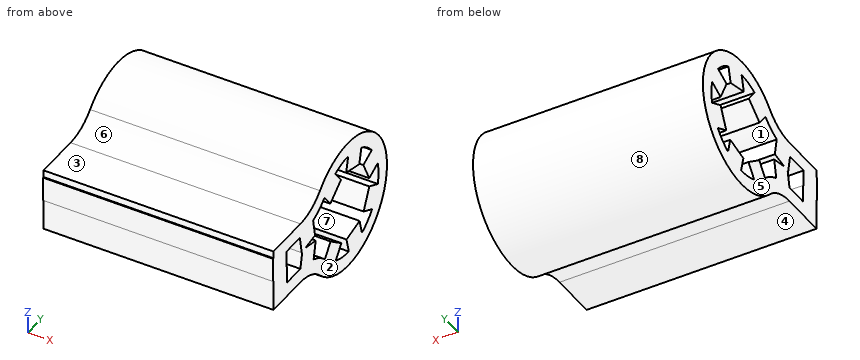
```python
from build123d import *

# Parameters (mm, degrees)
BOSS_EXTRUDE1_DEPTH = 5
BOSS_EXTRUDE2_DEPTH = 10
CRVPATTERN1_START   = -5
CRVPATTERN1_DEPTH   = 10


# Read off the part's stored shape, not the designer's step: CrvPattern1
with BuildPart() as part:
    # Sketch1 → Boss-Extrude1 (new, symmetric)
    with BuildSketch(Plane(origin=(0, 0, 0), x_dir=(0, 0, -1), z_dir=(1, 0, 0))):
        with BuildLine():
            Line((-0.74, -4.899518381), (-0.74, -3.529518381))
            ThreePointArc((-0.74, -3.529518381), (-0.951991552, -2.495045015), (-1.553790984, -1.627339417))
            ThreePointArc((-1.553790984, -1.627339417), (0, 2.25), (1.553790984, -1.627339417))
            ThreePointArc((1.553790984, -1.627339417), (0.951991552, -2.495045015), (0.74, -3.529518381))
            Line((0.74, -3.529518381), (0.74, -4.899518381))
            Line((0.74, -4.899518381), (0.74, -5.529518381))
            Line((0.74, -5.529518381), (1.37, -5.529518381))
            Line((1.37, -5.529518381), (1.37, -3.529518381))
            ThreePointArc((1.37, -3.529518381), (1.531210305, -2.74284662), (1.988852459, -2.082994454))
            ThreePointArc((1.988852459, -2.082994454), (0, 2.88), (-1.988852459, -2.082994454))
            ThreePointArc((-1.988852459, -2.082994454), (-1.531210305, -2.74284662), (-1.37, -3.529518381))
            Line((-1.37, -3.529518381), (-1.37, -5.529518381))
            Line((-1.37, -5.529518381), (-0.74, -5.529518381))
            Line((-0.74, -5.529518381), (-0.74, -4.899518381))
        make_face()
    extrude(amount=BOSS_EXTRUDE1_DEPTH, both=True)

    # Sketch2 → Boss-Extrude2 (add)
    with BuildSketch(Plane(origin=(5, 0, 0), x_dir=(0, 0, -1), z_dir=(1, 0, 0))):
        Polygon((0.74, -5.529518381), (-0.01, -5.529518381), (-0.01, -4.529518381), (1.055, -4.529518381), (1.055, -5.529518381), align=None)
    extrude(amount=-BOSS_EXTRUDE2_DEPTH)

    # CrvPattern1 outline → CrvPattern1 (add)
    with BuildSketch(Plane.YZ.offset(CRVPATTERN1_START)):
        with BuildLine():
            Line((-3.434132874, -0.045450425), (-3.397683617, -0.03901399))
            Line((-3.397683617, -0.03901399), (-3.532580052, -0.74))
            Line((-3.532580052, -0.74), (-3.529518381, -0.74))
            ThreePointArc((-3.529518381, -0.74), (-3.03102155, -0.78767529), (-2.550597709, -0.928972692))
            Line((-2.550597709, -0.928972692), (-2.399805364, -0.145383976))
            Line((-2.399805364, -0.145383976), (-3.165558429, 0.00197611))
            Line((-3.165558429, 0.00197611), (-2.449368801, 0.128445298))
            Line((-2.449368801, 0.128445298), (-2.588131662, 0.914253465))
            ThreePointArc((-2.588131662, 0.914253465), (-3.050829227, 0.783930261), (-3.529518381, 0.74))
            Line((-3.529518381, 0.74), (-3.572832561, 0.74))
            Line((-3.572832561, 0.74), (-3.434132874, -0.045450425))
        make_face()
        Polygon((-4.569835686, 0.01), (-4.569835686, 0.74), (-5.529518381, 0.74), (-5.529518381, 1.055), (-5.569835686, 1.055), (-5.569835686, -0.01), (-5.529518381, -0.01), (-5.529518381, 0.01), align=None)
        with BuildLine():
            Line((-1.299068151, -0.901344517), (-1.718974467, -1.462428052))
            ThreePointArc((-1.718974467, -1.462428052), (-1.672594961, -1.507545863), (-1.627339417, -1.553790984))
            ThreePointArc((-1.627339417, -1.553790984), (-1.295295274, -1.839758178), (-0.914118043, -2.055939737))
            Line((-0.914118043, -2.055939737), (-0.498447811, -1.500516504))
            Line((-0.498447811, -1.500516504), (-1.299068151, -0.901344517))
        make_face()
        with BuildLine():
            ThreePointArc((-1.627339417, 1.553790984), (-1.686697501, 1.493590875), (-1.747959826, 1.435329714))
            Line((-1.747959826, 1.435329714), (-1.315009752, 0.877923318))
            Line((-1.315009752, 0.877923318), (-0.525253811, 1.491344505))
            Line((-0.525253811, 1.491344505), (-0.950809299, 2.039230658))
            ThreePointArc((-0.950809299, 2.039230658), (-1.311726198, 1.828079424), (-1.627339417, 1.553790984))
        make_face()
        with BuildLine():
            Line((-0.118991671, -1.576654998), (0.050236755, -2.249439101))
            ThreePointArc((0.050236755, -2.249439101), (0.548855993, -2.182030499), (1.020028088, -2.005503104))
            Line((1.020028088, -2.005503104), (0.850799662, -1.332719001))
            Line((0.850799662, -1.332719001), (-0.118991671, -1.576654998))
        make_face()
        with BuildLine():
            ThreePointArc((0.983930045, 2.023457849), (0.509670601, 2.191514517), (0.009923593, 2.249978116))
            Line((0.009923593, 2.249978116), (-0.147222825, 1.574269812))
            Line((-0.147222825, 1.574269812), (0.826783627, 1.347749545))
            Line((0.826783627, 1.347749545), (0.983930045, 2.023457849))
        make_face()
        with BuildLine():
            Line((1.149073188, -1.086108101), (1.77806433, -1.378762938))
            ThreePointArc((1.77806433, -1.378762938), (2.03999745, -0.949163002), (2.199914553, -0.472097404))
            Line((2.199914553, -0.472097404), (1.570923411, -0.179442568))
            Line((1.570923411, -0.179442568), (1.149073188, -1.086108101))
        make_face()
        with BuildLine():
            ThreePointArc((2.191102417, 0.511439339), (2.022663, 0.98556298), (1.753074426, 1.410400673))
            Line((1.753074426, 1.410400673), (1.129428004, 1.106522654))
            Line((1.129428004, 1.106522654), (1.567455996, 0.20756132))
            Line((1.567455996, 0.20756132), (2.191102417, 0.511439339))
        make_face()
    extrude(amount=CRVPATTERN1_DEPTH)


solid = part.part
```
Model file for the job. Use its own axes, mm. Face numbers are marked on the shaded views. A direction names the side the tool comes from. Give positions to 0.01 mm unless a question says otherwise; leave off trailing zeros. Loops run counter-clockwise (first coordinate to the right, second up) from the corner with the lowest first, then second, coordinate; pieces in that order, holes last. Notation, with made-up numbers: (62, -17) -> (85, -17) arc R18 cw to (85, 13) -> close; hole circle Ø1 at (73, -40). An arc over 180 degrees is marked (long way). Use CSV: the item, a comma, the result in double quotes. Start each with the question number.
1) Wall check: line 1 (Z direction, x = 1, y = 1.25); line 2 (Y direction, x = 3, z = -0.55); line 3 (Y direction, x = 0.75, z = 0.3). Give the ranges that are in metal, low to high.
2) Slice it at A-A on y = -1.5. Give the cut face in (x, z).
3) Slice it at B-B on z = 0.35. Give the cut face in (x, y), plus the area to 3 significant figures.
4) Flat gauge pins, fed straight in: pin 1 Ø0.5 at (x, y) = (-2.5, -4) entering from +Z; pin 2 Ø1 at (x, z) = (-1.5, 1) entering from +Y; pin 3 Ø0.8 at (x, y) = (-2, -4) entering from -Z. Where does each tip first touch, or does it go through?
5) Slice it at C-C on x = -2.75. Give the number of separate pieces and of enclosed holes in the cut face, plus the area to 3 significant figures.
6) Tool access for the marked faces 1, 2, 3, 4 and 5: list every direction of +Z, -Z, +X, -X, +Y, -Y with a clear straight run to the whole face (end or side of a thin tool).
7) Mould opens along Y. For the marked faces 6, 7 and 8 say: released by +Y, released by -Y, zero draft, split by the parting line, or undercut.
8) Slice it at D-D on y = 0.5. Give the cut face in (x, z).
Computed values:
1,line 1,"z = -2.59 to -1.87, -1.13 to -0.87, 0.86 to 1.17, 1.87 to 2.59"
1,line 2,"y = -5.53 to -4.53, -3.5 to -2.48, 1.4 to 2.83"
1,line 3,"y = -5.57 to -4.57, -3.5 to -2.48, 1.52 to 1.76, 2.23 to 2.86"
2,outline,"(-5, -2.46) -> (5, -2.46) -> (5, -1.17) -> (-5, -1.17) -> close; (-5, 1.12) -> (5, 1.12) -> (5, 2.46) -> (-5, 2.46) -> close"
3,outline,"(-5, -5.57) -> (5, -5.57) -> (5, -4.57) -> (-5, -4.57) -> close; (-5, -3.5) -> (5, -3.5) -> (5, -2.49) -> (-5, -2.49) -> close; (-5, 1.5) -> (5, 1.5) -> (5, 1.86) -> (-5, 1.86) -> close; (-5, 2.22) -> (5, 2.22) -> (5, 2.86) -> (-5, 2.86) -> close"
3,area,"30.1 mm^2"
4,pin 1,"stops at z = 1.37"
4,pin 2,"stops at y = 2.84"
4,pin 3,"stops at z = -1.37"
5,separate pieces,"1"
5,enclosed holes,"2"
5,area,"20.0 mm^2"
6,face 1,"+X, -X"
6,face 2,"+Z, -Z, +X, +Y, -Y"
6,face 3,"+Z, +X, -X, -Y"
6,face 4,"-Z, +X, -X, -Y"
6,face 5,"+Z, -Z, -X, +Y, -Y"
7,face 6,"released by -Y"
7,face 7,"undercut"
7,face 8,"split by the parting line"
8,outline,"(-5, -2.84) -> (5, -2.84) -> (5, -1.42) -> (-5, -1.42) -> close; (-5, 1.42) -> (5, 1.42) -> (5, 2.84) -> (-5, 2.84) -> close"
